Could you check a few things on this model? Use its own coordinates, in mm. A direction names the side the tool comes from. Round coordinates to 2 decimals unless told otherwise and drop trailing zeros. Loops run counter-clockwise (first coordinate to the right, second up) from the corner with the lowest first, then second, coordinate; pieces in that order, holes last. Notation, with made-up numbers: (87.5, -9.75) -> (125.5, -9.75) arc R13 ccw to (125.5, 5.25) -> close; hole circle Ø10 at (-14.75, 66). An arc over 180 degrees is marked (long way). One line per item, written item: value.
Autodesk Fusion 360 part; units mm, degrees
sketch "Skizze1" plane through (0, 0, 0) normal (0, 1, 0) x (1, 0, 0)
  line L0 (9.5, 9.5) -> (-9.5, 9.5)
  line L1 (-9.5, 9.5) -> (-9.5, -9.5)
  line L2 (-9.5, -9.5) -> (9.5, -9.5)
  line L3 (9.5, -9.5) -> (9.5, 9.5)
  line L4 (9.5, 9.5) -> (-9.5, -9.5) construction
  line L5 (-9.5, 9.5) -> (9.5, -9.5) construction
  line L6 (4.5, 4.5) -> (-4.5, 4.5)
  line L7 (-4.5, 4.5) -> (-4.5, -4.5)
  line L8 (-4.5, -4.5) -> (4.5, -4.5)
  line L9 (4.5, -4.5) -> (4.5, 4.5)
  line L10 (4.5, 4.5) -> (-4.5, -4.5) construction
  line L11 (-4.5, 4.5) -> (4.5, -4.5) construction
  dimension "d1" = 19
  dimension "d2" = 19
  dimension "d3" = 9
  dimension "d4" = 9
extrude "Extrusion1" add sketch "Skizze1" along normal blind 50 contours L0 L1 L2 L3 | L6 L7 L8 L9 makes body 1
ref_plane "Arbeitsebene1" through (0, 25, 0) normal (1, 0, 0) x (0, 0, -1)
sketch "Skizze2" plane through (0, 25, 0) normal (1, 0, 0) x (0, 0, -1)
  line L0 (-9.5, 25) -> (9.5, 25)
  line L1 (9.5, 25) -> (9.5, 44)
  line L2 (9.5, 44) -> (-9.5, 44)
  line L3 (-9.5, 44) -> (-9.5, 25)
  dimension "d8" = 19
  dimension "d9" = 19
extrude "Extrusion2" add sketch "Skizze2" along normal mid plane 50 bodies 1
extrude "Extrusion3" cut sketch "Skizze1" along normal blind 10 contours L6 L7 L8 L9 bodies 1
copy_body "Körper->Berechn1" bodies 1 removing the originals makes body 2 in component "T-Griff"
component "T-Griff" placed x (1, 0, 0) y (0, 1, 0) z (0, 0, 1) at (0, 0, 0)
(1) If we section it at B-B, the plane x = -2.5: Please give me the cut outline in (y, z), then the cut area to 3 significant figures.
Recorded:
outline: (0, -9.5) -> (69, -9.5) -> (69, 9.5) -> (0, 9.5) -> (0, 4.5) -> (10, 4.5) -> (10, -4.5) -> (0, -4.5) -> close
area: 1,220 mm²
(2) If we section it at A-A, the plane y = 8: Please give me the cut outline in (x, z).
Recorded:
outline: (-9.5, -9.5) -> (9.5, -9.5) -> (9.5, 9.5) -> (-9.5, 9.5) -> close; hole (-4.5, -4.5) -> (4.5, -4.5) -> (4.5, 4.5) -> (-4.5, 4.5) -> close
(3) If we section it at D-D, the plane y = 46: Please give me the cut outline in (x, z).
Recorded:
outline: (-9.5, -9.5) -> (9.5, -9.5) -> (9.5, 9.5) -> (-9.5, 9.5) -> close
(4) For faces 1 (the face through (4.5, 5, 0)), 2 (the face through (9.5, 25, 0)), 3 (the face through (-9.5, 25, 0)), which set-ups out of +Z, -Z, +X, -X, +Y, -Y let a thin tool reach every point of the face, with its end or its side?
Recorded:
face 1: -Y
face 2: +Z, -Z, +X, -Y
face 3: +Z, -Z, -X, -Y
(5) Thinking about a two-plate mould opening in X: for faces 4 (the face through (0, 0, -6)), 5 (the face through (25, 60, 0)), 6 (the face through (0, 5, 4.5)), which applies, released by +X, released by -X, zero draft, split by the parting line, or undercut?
Recorded:
face 4: zero draft
face 5: released by +X
face 6: undercut
(6) If we section it at C-C, the plane z = 5.5: Please give me the cut outline in (x, y), then the cut area to 3 significant figures.
Recorded:
outline: (-25, 50) -> (-9.5, 50) -> (-9.5, 0) -> (9.5, 0) -> (9.5, 50) -> (25, 50) -> (25, 69) -> (-25, 69) -> close
area: 1,900 mm²
(7) If I drill on L1, parallel to Y at x = 16, z = -1.5; L2, parallel to X at y = 29, z = -4.5, over which ranges is the centre line in solid material (lowest first)?
Recorded:
L1: 50 to 69
L2: -9.5 to 9.5
(8) I'm going to push flat-ended pins straight in: pin 1 Ø2.5 at (y, z) = (7, 0) entering from -X; pin 2 Ø10 at (y, z) = (6, -0.5) entering from +X; pin 3 Ø12 at (x, y) = (-18.5, 7.5) entering from -Z; pin 4 Ø8 at (x, z) = (14, 3.5) entering from -Y. Where does each tip first touch, or does it pass through?
Recorded:
pin 1: x = -9.5
pin 2: x = 9.5
pin 3: through
pin 4: y = 50
